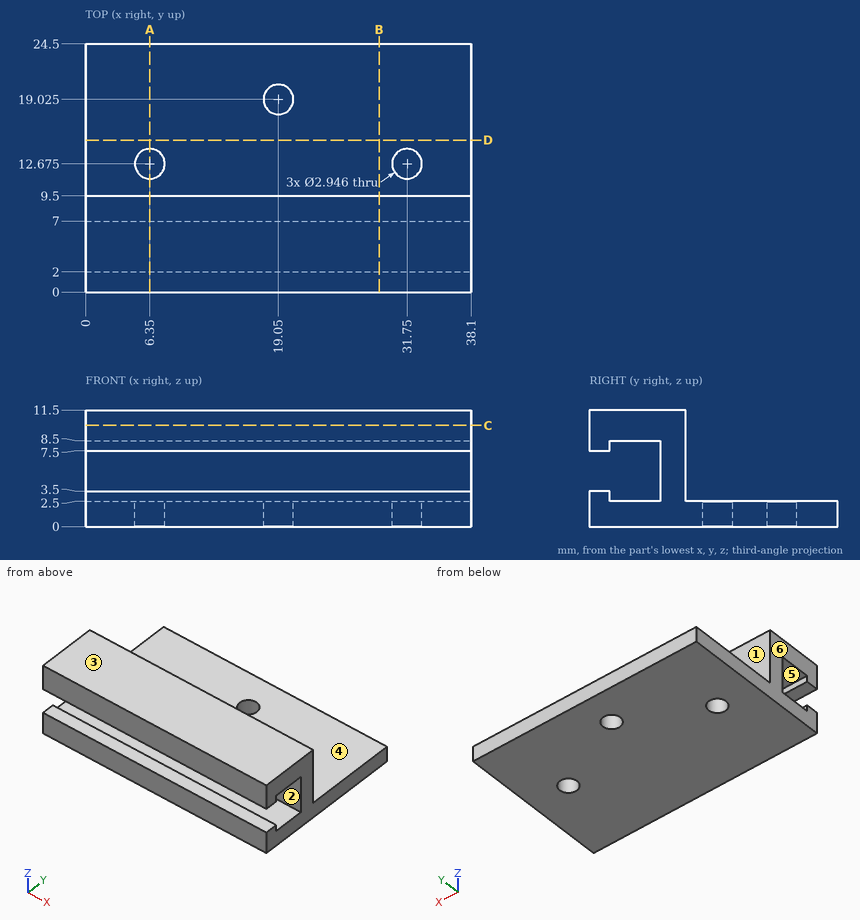
Source: three-view drawing plus pictorial views. Frame: mm from the lowest corner of the part. A direction names the side the tool comes from. Give positions to 0.01 mm unless a question says otherwise; leave off trailing zeros. Order: outer loops, then holes, each group sorted by start corner. A loop starts at its lowest first (then second) coordinate and runs counter-clockwise, first axis right, second up. Notation, with made-up numbers: (76, -27.5) - (94, -27.5) arc R13 cw to (94, -14.5) - close; hole circle Ø1 at (-2, 2). An arc over 180 degrees is marked (long way). Put each result on its own line as item: value.
Item 1: Section query B-B, the plane x = 29. Return loops of the section in (y, z), then the cut area to 3 significant figures.
Found:
outline: (0, 0) - (24.5, 0) - (24.5, 2.5) - (9.5, 2.5) - (9.5, 11.5) - (0, 11.5) - (0, 7.5) - (2, 7.5) - (2, 8.5) - (7, 8.5) - (7, 2.5) - (2, 2.5) - (2, 3.5) - (0, 3.5) - close
area: 109 mm^2
Item 2: Ray query, L1, parallel to Y at x = 31.75, z = 1; L2, parallel to Z at x = 20.5, y = 6; L3, parallel to Z at x = 20, y = 14.5. Return the intervals inside material, ascending. Write a range as from..to.
Found:
L1: y = 0..11.2, 14.15..24.5
L2: z = 0..2.5, 8.5..11.5
L3: z = 0..2.5
Item 3: Access query for the marked faces 1, 2 and 3. Directions: +Z, -Z, +X, -X, +Y, -Y. A direction counts if a zero-diameter tool reaches every point of the face in a straight line with its end or side. Return the directions, or none.
Found:
face 1: +Z, +X, -X, +Y
face 2: +X, -X
face 3: +Z, +X, -X, +Y, -Y
Item 4: Section query C-C, the plane z = 10. Return loops of the section in (x, y), then the cut area to 3 significant figures.
Found:
outline: (0, 0) - (38.1, 0) - (38.1, 9.5) - (0, 9.5) - close
area: 362 mm^2
Item 5: Section query D-D, the plane y = 15. Return loops of the section in (x, z).
Found:
outline: (0, 0) - (38.1, 0) - (38.1, 2.5) - (0, 2.5) - close
Item 6: Contact query for flat-ended pins moving along their axis: pin 1 (1 mm diameter, centred on x = 10.5, y = 16, fed in from +Z); pin 2 (2.5 mm diameter, centred on x = 23.5, z = 6.5, fed in from +Y); pin 3 (3 mm diameter, centred on x = 30, z = 5.5, fed in from -Y). Output: stop coordinate, or through.
Found:
pin 1: stops at z = 2.5
pin 2: stops at y = 9.5
pin 3: stops at y = 7
Item 7: Draft query along Z for the marked faces 4, 5 and 6. Return one class per face: +Z half, -Z half, draft (parallel to the pull), parting line (faces both ways), or undercut.
Found:
face 4: +Z half
face 5: undercut
face 6: draft
Item 8: Section query A-A, the plane x = 6.35. Return loops of the section in (y, z).
Found:
outline: (0, 0) - (11.2, 0) - (11.2, 2.5) - (9.5, 2.5) - (9.5, 11.5) - (0, 11.5) - (0, 7.5) - (2, 7.5) - (2, 8.5) - (7, 8.5) - (7, 2.5) - (2, 2.5) - (2, 3.5) - (0, 3.5) - close; (14.15, 0) - (24.5, 0) - (24.5, 2.5) - (14.15, 2.5) - close
